Check sheet for the modelled part. Datum: model origin and axes. Units: mm. A direction names the side the tool comes from. Give positions to 0.01 mm unless a question says otherwise; leave off trailing zeros. Order: outer loops, then holes, each group sorted by start corner. A loop starts at its lowest first (then second) coordinate and runs counter-clockwise, first axis right, second up. Notation, with made-up numbers: M -8,76.5 L 37,76.5 A24 cw 37,109.5 Z; hole C 89.5,73 d6. An arc over 180 degrees is marked long. Answer in a Markdown table with one row per item. Add a question column.
from build123d import *

# Parameters (mm, degrees)
CROQUIS1_R              = 19
CROQUIS1_R_2            = 1.5
SALIENTE_EXTRUIR1_DEPTH = 1.5
SALIENTE_EXTRUIR2_DEPTH = 14
SALIENTE_EXTRUIR3_START = 10
CROQUIS3_R              = 19
CROQUIS3_R_2            = 3
SALIENTE_EXTRUIR3_DEPTH = 10


with BuildPart() as part:
    # Croquis1 → Saliente-Extruir1 (new body)
    with BuildSketch(Plane.XY):
        with Locations((-84.957007, 9.639802)):
            Circle(CROQUIS1_R)
        with Locations((-84.957007, 19.139802)):
            Circle(CROQUIS1_R_2, mode=Mode.SUBTRACT)
        with Locations((-92.957007, 9.639802)):
            Circle(CROQUIS1_R_2, mode=Mode.SUBTRACT)
        with Locations((-84.957007, 0.139802)):
            Circle(CROQUIS1_R_2, mode=Mode.SUBTRACT)
        with Locations((-76.957007, 9.639802)):
            Circle(CROQUIS1_R_2, mode=Mode.SUBTRACT)
    extrude(amount=SALIENTE_EXTRUIR1_DEPTH)

    # Croquis2 → Saliente-Extruir2 (add)
    with BuildSketch(Plane.XY.offset(1.5)):
        with BuildLine():
            Line((-98.392036, 23.074831), (-96.977823, 21.660617))
            ThreePointArc((-96.977823, 21.660617), (-72.936192, 21.660617), (-72.936192, -2.381013))
            Line((-72.936192, -2.381013), (-71.521978, -3.795227))
            ThreePointArc((-71.521978, -3.795227), (-71.521978, 23.074831), (-98.392036, 23.074831))
        make_face()
    extrude(amount=SALIENTE_EXTRUIR2_DEPTH)

    # Croquis3 → Saliente-Extruir3 (add)
    with BuildSketch(Plane(origin=(0, 0, 0), x_dir=(-1, 0, 0), z_dir=(0, 0, -1)).offset(SALIENTE_EXTRUIR3_START)):
        with Locations((84.957007, 9.639802)):
            Circle(CROQUIS3_R)
        with Locations((84.957007, 0.139802)):
            Circle(CROQUIS3_R_2, mode=Mode.SUBTRACT)
        with Locations((76.957007, 9.639802)):
            Circle(CROQUIS3_R_2, mode=Mode.SUBTRACT)
        with Locations((92.957007, 9.639802)):
            Circle(CROQUIS3_R_2, mode=Mode.SUBTRACT)
        with Locations((84.957007, 19.139802)):
            Circle(CROQUIS3_R_2, mode=Mode.SUBTRACT)
    extrude(amount=-SALIENTE_EXTRUIR3_DEPTH)

    # Croquis5 → Cortar-Revolución1 (revolve, cut)
    with BuildSketch(Plane(origin=(0, 9.639802, 0), x_dir=(-1, 0, 0), z_dir=(0, -1, 0)), mode=Mode.PRIVATE) as cortar_revoluci_n1_sk:
        Polygon((90.957007, 10), (103.957007, 0), (103.957007, 10), align=None)
    revolve(cortar_revoluci_n1_sk.sketch.rotate(Axis((-84.957007, 9.639802, 0), (0, 0, -1)), 45), axis=Axis((-84.957007, 9.639802, 0), (0, 0, -1)), mode=Mode.SUBTRACT)


solid = part.part
Q1. Go/stop test with flat-tipped pins: pin 1 (9.5 mm diameter, centred on x = -92.96, y = 9.64, fed in from +Z); pin 2 (10 mm diameter, centred on x = -95.5, y = 17, fed in from +Z); pin 3 (2.5 mm diameter, centred on x = -84.96, y = 0.14, fed in from +Z); pin 4 (5 mm diameter, centred on x = -90.5, z = 2.5, fed in from +Y). Record where each tip stops, or that it passes through.
Q2. Tool access check on faces 4 (the flat face through (-72.24, -3.08, 8.4)), 5 (the flat face through (-73, 22, 15.5)), 6 (the flat face through (-84, 21, 0)). Record the directions out of +Z, -Z, +X, -X, +Y, -Y that give a thin tool (end or side, any length) a straight path to the whole face; none if there is none.
Q3. Cross-section at A-A (z = -3.75). Record the boundary of the cut face in (x, y) (3 decimals), and give its area (3 significant figures).
Q4. Thickness scan on probe 1 along Y at (x, z) = (-94, -2.5); probe 2 along X at (y, z) = (1.5, -4); probe 3 along Y at (x, z) = (-85, 3.25). Record the ranges inside material, lowest first.
Q5. Cross-section at C-C (z = -0.5). Record the boundary of the cut face in (x, y).
Q6. Draft check along X on faces 1 (the conical face through (-88.105, 15.682, -9.374)), 2 (the flat face through (-85, 10, -10)), 3 (the cylindrical face through (-91.526, 10.09, 0.74)). Enter one of: pulls with the +X half, pulls with the -X half, needs draft (parallel to the pull), parting line crosses it, or undercut.
Values follow:
| question | item | result |
|---|---|---|
| 1 | pin 1 | z = 1.5 |
| 1 | pin 2 | z = 15.5 |
| 1 | pin 3 | through |
| 1 | pin 4 | y = 28.39 |
| 2 | face 4 | +Z, -X, -Y |
| 2 | face 5 | +Z, +X, -X, +Y, -Y |
| 2 | face 6 | -Z |
| 3 | outline | C -84.957,9.64 d28.25; hole C -92.957,9.64 d6; hole C -84.957,0.14 d6; hole C -84.957,19.14 d6; hole C -76.957,9.64 d6 |
| 3 | area | 514 mm² |
| 4 | probe 1 | -3.26 to 6.83, 12.45 to 22.54 |
| 4 | probe 2 | -96.1 to -87.63, -82.28 to -73.81 |
| 4 | probe 3 | 26.64 to 28.64 |
| 5 | outline | C -84.96,9.64 d36.7; hole C -92.96,9.64 d6; hole C -84.96,0.14 d6; hole C -84.96,19.14 d6; hole C -76.96,9.64 d6 |
| 6 | face 1 | parting line crosses it |
| 6 | face 2 | needs draft |
| 6 | face 3 | undercut |
